The model under review builds one solid part; all positions refer to its coordinate system, in mm. A direction names the side the tool comes from. Give positions to 0.01 mm unless a question says otherwise; leave off trailing zeros. Order: outer loops, then holes, each group sorted by start corner. A loop starts at its lowest first (then second) coordinate and runs counter-clockwise, first axis right, second up. Notation, with made-up numbers: (8, -24.75) -> (50, -24.75) arc R34 ccw to (50, 6.25) -> close; hole circle Ø4 at (-24, -25). An arc over 180 degrees is marked (long way). Answer as a JSON object with one key per item and string values. Group by question number.
Autodesk Inventor part; units mm, degrees
ref_plane "YZ Plane" through (0, 0, 0) normal (1, 0, 0) x (0, 1, 0)
ref_plane "XZ Plane" through (0, 0, 0) normal (0, 1, 0) x (-1, 0, 0)
ref_plane "XY Plane" through (0, 0, 0) normal (0, 0, 1) x (1, 0, 0)
sketch "Sketch1" plane through (0, 0, 0) normal (0, 0, 1) x (1, 0, 0)
  line L0 (-48.8512, -88.9904) -> (65.4488, -88.9904)
  line L1 (65.4488, -88.9904) -> (65.4488, 23.9678)
  line L2 (64.4867, 26.2447) -> (10.5117, 78.7012)
  line L3 (6.086, 78.7012) -> (-47.889, 26.2447)
  line L4 (-48.8512, 23.9678) -> (-48.8512, -88.9904)
  circle A0 centre (8.2988, 63.4096) radius 3.175
  arc A1 (10.5117, 78.7012) -> (6.086, 78.7012) centre (8.2988, 76.4243) ccw
  arc A2 (-47.889, 26.2447) -> (-48.8512, 23.9678) centre (-45.6762, 23.9678) ccw
  arc A3 (65.4488, 23.9678) -> (64.4867, 26.2447) centre (62.2738, 23.9678) ccw
  point P0 (0, 0)
  point P1 (65.4488, 25.3096)
  point P2 (8.2988, 80.8517)
  point P3 (-48.8512, 25.3096)
  dimension "d0" = 114.3
  dimension "d1" = 114.3
  dimension "d2" = 114.3
  dimension "d3" = 57.15
  dimension "d4" = 6.35
  dimension "d5" = 152.4
  dimension "d6" = 3.175
  dimension "d29" = 57.15
extrude "Extrusion1" add sketch "Sketch1" against normal blind 6.35
sketch "Sketch2" plane through (0, 0, 0) normal (0, 0, 1) x (1, 0, 0)
  line L0 (65.4488, -88.9904) -> (-48.8512, -88.9904)
  line L1 (-48.8512, -88.9904) -> (65.4488, -88.9904)
  line L2 (65.4488, -88.9904) -> (65.4488, -82.6404)
  line L3 (65.4488, -82.6404) -> (-48.8512, -82.6404)
  line L4 (-48.8512, -82.6404) -> (-48.8512, -88.9904)
  point P0 (0, 0)
  dimension "d9" = 6.35
  dimension "d30" = 114.3
extrude "Extrusion2" add sketch "Sketch2" along normal blind 144.4498
hole "Hole1" at (-29.8012, -82.6404, 131.7498) direction (0, -1, 0) diameter 6.35 end through all
pattern_linear "Rectangular Pattern1" count 2 spacing 63.5 along (0, 0, -1) count 2 spacing 76.2 along (1, 0, 0) of "Hole1"
properties part number "Braquet Rammasse-Balle"
1. Machinability: for faces 1 (the flat face through (9, -82.64, 71)), 2 (the flat face through (7, -22, -6.35)), which of the approach directions +Z, -Z, +X, -X, +Y, -Y give a long, thin tool a straight path to every point of the face, cutting with its end or side? Answer none if there is none.
2. Take a section at D-D on x = 52. Give the boundary of the cut face in (y, z).
3. For probe 1 along Z at (x, y) = (-28, -64.5); probe 2 along Y at (x, z) = (-12, 23.5), list the stretches that pass through material, from the lowest coordinate up. Write a range as [from, to].
4. For pin 1 (4 mm diameter, centred on x = 8.3, y = 63.41, fed in from -Z); pin 2 (8 mm diameter, centred on x = 17, y = 34, fed in from +Z); pin 3 (6 mm diameter, centred on x = 6.5, z = 82.5, fed in from +Y), all flat-tipped, find the tip position at first contact; note any pin that passes through.
5. Draft analysis for pull direction Z (two halves, no side actions). For faces 3 (the cylindrical face through (48.33, -85.86, 65.73)), 4 (the cylindrical face through (8.3, 79.6, -3.1)), 5 (the flat face through (7, -86, 144.45)), state which applies: pulls with the +Z half, pulls with the -Z half, needs draft (parallel to the pull), parting line crosses it, or undercut.
6. Take a section at B-B on y = 19. Give the boundary of the cut face in (x, z).
7. Take a section at C-C on z = 36.5. Give the boundary of the cut face in (x, y), plus the area to 3 significant figures.
8. Take a section at A-A on x = -17. Give the boundary of the cut face in (y, z), plus the area to 3 significant figures.
Checks:
{
 "1": {"face 1": "+Z, +X, -X, +Y", "face 2": "-Z, +X, -X, +Y, -Y"},
 "2": {"outline": "(-88.99, -6.35) -> (38.38, -6.35) -> (38.38, 0) -> (-82.64, 0) -> (-82.64, 144.45) -> (-88.99, 144.45) -> close"},
 "3": {"probe 1": "z = [-6.35, 0]", "probe 2": "y = [-88.99, -82.64]"},
 "4": {"pin 1": "passes through", "pin 2": "stops at z = 0", "pin 3": "stops at y = -82.64"},
 "5": {"face 3": "undercut", "face 4": "needs draft", "face 5": "pulls with the +Z half"},
 "6": {"outline": "(-48.85, -6.35) -> (65.45, -6.35) -> (65.45, 0) -> (-48.85, 0) -> close"},
 "7": {"outline": "(-48.85, -88.99) -> (65.45, -88.99) -> (65.45, -82.64) -> (-48.85, -82.64) -> close", "area": "726 mm2"},
 "8": {"outline": "(-88.99, -6.35) -> (56.26, -6.35) -> (56.26, 0) -> (-82.64, 0) -> (-82.64, 144.45) -> (-88.99, 144.45) -> close", "area": "1,840 mm2"}
}
